Can you work these out from the model? Positions are in its coordinate system, mm. Face numbers are marked on the shaded views. A direction names the side the tool comes from. Give positions to 0.01 mm unless a question says otherwise; leave off trailing zeros. Write each loop counter-clockwise with the first axis right and the second up, starting at its lowest first coordinate (ties: lowest second). Pieces come first, ordered by that corner, then holes. Notation, with made-up numbers: (56.5, -21) -> (65.5, -21) arc R32 cw to (65.5, 6) -> close; hole circle Ø7 at (35.5, -20). An arc over 180 degrees is marked (long way). One line per item, written item: value.
from build123d import *

# Parameters (mm, degrees)
F0_W         = 76.2
F0_H         = 152.4
F0_W_2       = 67.8425729275
F0_H_2       = 3.318388015
F0_H_3       = 2.9496736825
F1_DEPTH     = 50.8
F2_W         = 76.2
F2_H         = 152.4
F2_W_2       = 67.8425729275
F2_H_2       = 15.301451087
F2_H_3       = 89.0433862805
F2_H_4       = 31.7090302706
F3_DEPTH     = 5.08
F4_T1_DEPTH  = 81.28
F4_T3_DEPTH  = 177.8
F5_T1_DEPTH  = 66.04
F5_S5_W      = 5.08
F5_S5_H      = 5.08
F5_T6_DEPTH  = 5.08
F5_S11_W     = 5.08
F5_S11_H     = 5.08
F5_T12_DEPTH = 5.08
F6_T1_DEPTH  = 160.02
F6_T3_DEPTH  = 66.04
F6_S7_W      = 5.08
F6_S7_H      = 5.08
F6_T8_DEPTH  = 5.08
F6_T12_ANGLE = 89.9999999979
F7_W         = 67.8425729275
F7_H         = 4.4245161116
F8_DEPTH     = 50.8
F9_R         = 14.2326914524
F10_DEPTH    = 25.4


# Not quite as in the source:
# - a fillet or chamfer that OpenCascade refuses, or shapes differently, is made with other operations: its cross-section is extruded or revolved along the edge and cut away or added


with BuildPart() as f1:
    # F0 (on Front) → F1 (new body)
    with BuildSketch(Plane.XZ):
        Rectangle(F0_W, F0_H)
        Polygon((-33.9212864637, 71.1609646678), (33.9212864637, 71.1609646678), (33.9212864637, 39.4519343972), (33.9212864637, 36.1335463822), (33.9212864637, -52.9098398983), (33.9212864637, -55.8595135808), (33.9212864637, -71.1609646678), (-33.9212864637, -71.1609646678), (-33.9212864637, -55.8595135808), (-33.9212864637, -52.9098398983), (-33.9212864637, 36.1335463822), (-33.9212864637, 39.4519343972), align=None, mode=Mode.SUBTRACT)
        with Locations((0, 37.7927403897)):
            Rectangle(F0_W_2, F0_H_2)
        with Locations((0, -54.3846767396)):
            Rectangle(F0_W_2, F0_H_3)
    extrude(amount=F1_DEPTH)

    # F2 (on face) → F3 (join)
    with BuildSketch(Plane(origin=(0, 0, 0), x_dir=(-1, 0, 0), z_dir=(0, 1, 0))):
        Rectangle(F2_W, F2_H)
        with Locations((0, -63.5102391243)):
            Rectangle(F2_W_2, F2_H_2, mode=Mode.SUBTRACT)
        with Locations((0, -8.3881467581)):
            Rectangle(F2_W_2, F2_H_3, mode=Mode.SUBTRACT)
        with Locations((0, 55.3064495325)):
            Rectangle(F2_W_2, F2_H_4, mode=Mode.SUBTRACT)
        with Locations((0, 55.3064495325)):
            Rectangle(F2_W_2, F2_H_4)
        with Locations((0, -63.5102391243)):
            Rectangle(F2_W_2, F2_H_2)
        with Locations((0, -8.3881467581)):
            Rectangle(F2_W_2, F2_H_3)
    extrude(amount=F3_DEPTH)

    # F4: fillet of radius 5.08 on 6 edges, made by hand

    # F4_s2 → F4_t1 (cut)
    with BuildSketch(Plane.XZ.offset(-17.78)):
        with BuildLine():
            ThreePointArc((38.1, -71.12), (36.6121024484, -74.7121024484), (33.02, -76.2))
            Line((33.02, -76.2), (38.1, -76.2))
            Line((38.1, -76.2), (38.1, -71.12))
        make_face()
        with BuildLine():
            ThreePointArc((38.1, 71.12), (36.6121024484, 74.7121024484), (33.02, 76.2))
            Line((33.02, 76.2), (38.1, 76.2))
            Line((38.1, 76.2), (38.1, 71.12))
        make_face()
        with BuildLine():
            ThreePointArc((-38.1, 71.12), (-36.6121024484, 74.7121024484), (-33.02, 76.2))
            Line((-33.02, 76.2), (-38.1, 76.2))
            Line((-38.1, 76.2), (-38.1, 71.12))
        make_face()
    extrude(amount=F4_T1_DEPTH, mode=Mode.SUBTRACT)

    # F4_s4 → F4_t3 (cut)
    with BuildSketch(Plane.XY.offset(-88.9)):
        with BuildLine():
            ThreePointArc((38.1, -45.72), (36.6121024484, -49.3121024484), (33.02, -50.8))
            Line((33.02, -50.8), (38.1, -50.8))
            Line((38.1, -50.8), (38.1, -45.72))
        make_face()
        with BuildLine():
            ThreePointArc((38.1, 0), (36.6121024484, 3.5921024484), (33.02, 5.08))
            Line((33.02, 5.08), (38.1, 5.08))
            Line((38.1, 5.08), (38.1, 0))
        make_face()
        with BuildLine():
            ThreePointArc((-33.02, 5.08), (-36.6121024484, 3.5921024484), (-38.1, 0))
            Line((-38.1, 0), (-38.1, 5.08))
            Line((-38.1, 5.08), (-33.02, 5.08))
        make_face()
    extrude(amount=F4_T3_DEPTH, mode=Mode.SUBTRACT)

    # F5: fillet of radius 5.08 on 1 edges, made by hand

    # F5_s2 → F5_t1 (cut)
    with BuildSketch(Plane.YZ.offset(-33.02)):
        with BuildLine():
            ThreePointArc((5.08, 71.12), (3.5921024484, 74.7121024484), (0, 76.2))
            Line((0, 76.2), (5.08, 76.2))
            Line((5.08, 76.2), (5.08, 71.12))
        make_face()
    extrude(amount=F5_T1_DEPTH, mode=Mode.SUBTRACT)


with BuildPart() as f5_tool4:
    # F5_s5 → F5_t6 (new body)
    with BuildSketch(Plane.XZ):
        with Locations((-35.56, 73.66)):
            Rectangle(F5_S5_W, F5_S5_H)
    extrude(amount=-F5_T6_DEPTH)

    # F5_s7 → F5_t8 (revolve, cut)
    with BuildSketch(Plane(origin=(-33.02, 0, 71.12), x_dir=(0.7071067812, 0, -0.7071067812), z_dir=(0.7071067812, 0, 0.7071067812))):
        with BuildLine():
            ThreePointArc((0, -5.08), (5.08, 0), (0, 5.08))
            Line((0, 5.08), (0, -5.08))
        make_face()
    revolve(axis=Axis((-33.02, 0, 71.12), (0, 1, 0)), mode=Mode.SUBTRACT)


with BuildPart() as f1_1:
    add(f1.part)

    # F5_t3: cut F5_tool4
    add(f5_tool4.part, mode=Mode.SUBTRACT)


with BuildPart() as f5_tool10:
    # F5_s11 → F5_t12 (new body)
    with BuildSketch(Plane.XZ):
        with Locations((35.56, 73.66)):
            Rectangle(F5_S11_W, F5_S11_H)
    extrude(amount=-F5_T12_DEPTH)

    # F5_s13 → F5_t14 (revolve, cut)
    with BuildSketch(Plane(origin=(33.02, 0, 71.12), x_dir=(-0.7071067812, 0, -0.7071067812), z_dir=(0.7071067812, 0, -0.7071067812))):
        with BuildLine():
            ThreePointArc((0, -5.08), (5.08, 0), (0, 5.08))
            Line((0, 5.08), (0, -5.08))
        make_face()
    revolve(axis=Axis((33.02, 0, 71.12), (0, 1, 0)), mode=Mode.SUBTRACT)


with BuildPart() as f1_2:
    add(f1_1.part)

    # F5_t9: cut F5_tool10
    add(f5_tool10.part, mode=Mode.SUBTRACT)

    # F6: fillet of radius 5.08 on 1 edges, made by hand

    # F6_s2 → F6_t1 (cut)
    with BuildSketch(Plane.XY.offset(-88.9)):
        with BuildLine():
            ThreePointArc((-33.02, -50.8), (-36.6121024484, -49.3121024484), (-38.1, -45.72))
            Line((-38.1, -45.72), (-38.1, -50.8))
            Line((-38.1, -50.8), (-33.02, -50.8))
        make_face()
    extrude(amount=F6_T1_DEPTH, mode=Mode.SUBTRACT)

    # F6_s4 → F6_t3 (cut)
    with BuildSketch(Plane.YZ.offset(-33.02)):
        with BuildLine():
            ThreePointArc((-45.72, 76.2), (-49.3121024484, 74.7121024484), (-50.8, 71.12))
            Line((-50.8, 71.12), (-50.8, 76.2))
            Line((-50.8, 76.2), (-45.72, 76.2))
        make_face()
    extrude(amount=F6_T3_DEPTH, mode=Mode.SUBTRACT)


with BuildPart() as f6_tool6:
    # F6_s7 → F6_t8 (new body)
    with BuildSketch(Plane.XY.offset(71.12)):
        with Locations((35.56, -48.26)):
            Rectangle(F6_S7_W, F6_S7_H)
    extrude(amount=F6_T8_DEPTH)

    # F6_s9 → F6_t10 (revolve, cut)
    with BuildSketch(Plane(origin=(33.02, -45.72, 71.12), x_dir=(-0.7071067812, 0.7071067812, 0), z_dir=(0.7071067812, 0.7071067812, 0))):
        with BuildLine():
            ThreePointArc((0, -5.08), (5.08, 0), (0, 5.08))
            Line((0, 5.08), (0, -5.08))
        make_face()
    revolve(axis=Axis((33.02, -45.72, 71.12), (0, 0, 1)), mode=Mode.SUBTRACT)


with BuildPart() as f1_3:
    add(f1_2.part)

    # F6_t5: cut F6_tool6
    add(f6_tool6.part, mode=Mode.SUBTRACT)

    # F6_s11 → F6_t12 (revolve, cut)
    with BuildSketch(Plane.XY.offset(71.1199999999)):
        with BuildLine():
            ThreePointArc((-33.02, -50.8), (-36.6121024484, -49.3121024484), (-38.1, -45.72))
            Line((-38.1, -45.72), (-38.1, -50.8))
            Line((-38.1, -50.8), (-33.02, -50.8))
        make_face()
    revolve(axis=Axis((-33.0199999999, -50.8, 71.1199999999), (0, 1, 0)), revolution_arc=F6_T12_ANGLE, mode=Mode.SUBTRACT)

    # F7 (on face) → F8 (join)
    with BuildSketch(Plane.XZ):
        Rectangle(F7_W, F7_H)
    extrude(amount=F8_DEPTH)

    # F9 (on face) → F10 (cut)
    with BuildSketch(Plane(origin=(0, 5.08, 0), x_dir=(-1, 0, 0), z_dir=(0, 1, 0))):
        with Locations((19.2330349237, -24.0364484489)):
            Circle(F9_R)
    extrude(amount=-F10_DEPTH, mode=Mode.SUBTRACT)


solid = f1_3.part
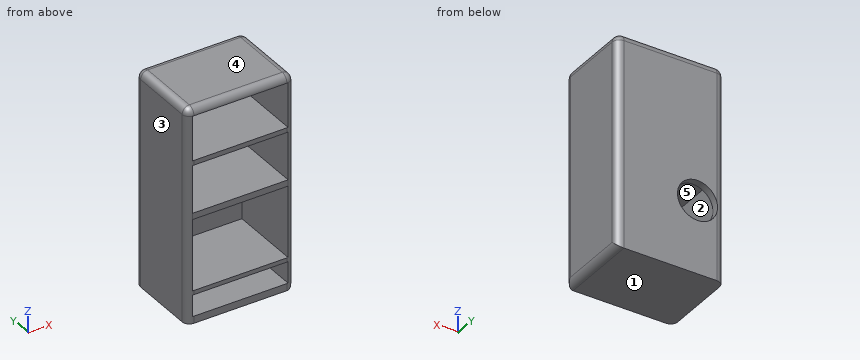
1) We'd pull the mould along Z, two halves only. Please class the marked faces 3, 4 and 5: released by +Z, released by -Z, zero draft, split by the parting line, or undercut.
Answer list:
face 3: zero draft
face 4: released by +Z
face 5: undercut
2) If we section it at C-C (x = 19): Write out the boundary of the cut face in (y, z), and give its area (3 significant figures).
Answer list:
outline: (-50.8, -76.2) -> (5.08, -76.2) -> (5.08, 71.12) arc R5.08 ccw to (0, 76.2) -> (-45.72, 76.2) arc R5.08 ccw to (-50.8, 71.16) -> (0, 71.16) -> (0, 39.45) -> (-50.8, 39.45) -> (-50.8, 36.13) -> (0, 36.13) -> (0, 2.21) -> (-50.8, 2.21) -> (-50.8, -2.21) -> (0, -2.21) -> (0, -52.91) -> (-50.8, -52.91) -> (-50.8, -55.86) -> (0, -55.86) -> (0, -71.16) -> (-50.8, -71.16) -> close
area: 1,820 mm^2
3) If we section it at A-A (x = -21.5): Write out the boundary of the cut face in (y, z), and give its area (3 significant figures).
Answer list:
outline: (-50.8, -76.2) -> (5.08, -76.2) -> (5.08, -38.09) -> (0, -38.09) -> (0, -52.91) -> (-50.8, -52.91) -> (-50.8, -55.86) -> (0, -55.86) -> (0, -71.16) -> (-50.8, -71.16) -> close; (-50.8, -2.21) -> (0, -2.21) -> (0, -9.99) -> (5.08, -9.99) -> (5.08, 71.12) arc R5.08 ccw to (0, 76.2) -> (-45.72, 76.2) arc R5.08 ccw to (-50.8, 71.16) -> (0, 71.16) -> (0, 39.45) -> (-50.8, 39.45) -> (-50.8, 36.13) -> (0, 36.13) -> (0, 2.21) -> (-50.8, 2.21) -> close
area: 1,680 mm^2
4) For the marked faces 1 and 2, which set-ups out of +Z, -Z, +X, -X, +Y, -Y let a thin tool reach every point of the face, with its end or its side?
Answer list:
face 1: -Z, +X, -X, +Y, -Y
face 2: -Y
5) I need wall thicknesses on L1, parallel to Z at x = -32.5, y = -14.5; L2, parallel to X at y = -14.5, z = -65.5; L3, parallel to Y at x = -16.5, z = 62. Which ranges of each line are inside material? Lowest first, please.
Answer list:
L1: z = -76.2 to -71.16, -55.86 to -52.91, -2.21 to 2.21, 36.13 to 39.45, 71.16 to 76.2
L2: x = -38.1 to -33.92, 33.92 to 38.1
L3: y = 0 to 5.08
6) If we section it at D-D (z = 33.5): Write out the boundary of the cut face in (x, y), and give its area (3 significant figures).
Answer list:
outline: (-38.1, -45.72) arc R5.08 ccw to (-33.92, -50.72) -> (-33.92, 0) -> (33.92, 0) -> (33.92, -50.72) arc R5.08 ccw to (38.1, -45.72) -> (38.1, 0) arc R5.08 ccw to (33.02, 5.08) -> (-33.02, 5.08) arc R5.08 ccw to (-38.1, 0) -> close
area: 790 mm^2
7) Will these pins go through, and if not, where does the flat tip stop? pin 1 (12 mm diameter, centred on x = 28, z = -36.5, fed in from -Y); pin 2 (8 mm diameter, centred on x = -20, z = 51.5, fed in from -Y).
Answer list:
pin 1: stops at y = -50.72
pin 2: stops at y = 0
8) If we section it at B-B (y = -21.5): Write out the boundary of the cut face in (x, z).
Answer list:
outline: (-38.1, -76.2) -> (33.02, -76.2) arc R5.08 ccw to (38.1, -71.12) -> (38.1, 71.12) arc R5.08 ccw to (33.02, 76.2) -> (-33.02, 76.2) arc R5.08 ccw to (-38.1, 71.12) -> close; hole (-33.92, -71.16) -> (33.92, -71.16) -> (33.92, -55.86) -> (-33.92, -55.86) -> close; hole (-33.92, -52.91) -> (33.92, -52.91) -> (33.92, -2.21) -> (-33.92, -2.21) -> close; hole (-33.92, 2.21) -> (33.92, 2.21) -> (33.92, 36.13) -> (-33.92, 36.13) -> close; hole (-33.92, 39.45) -> (33.92, 39.45) -> (33.92, 71.16) -> (-33.92, 71.16) -> close
